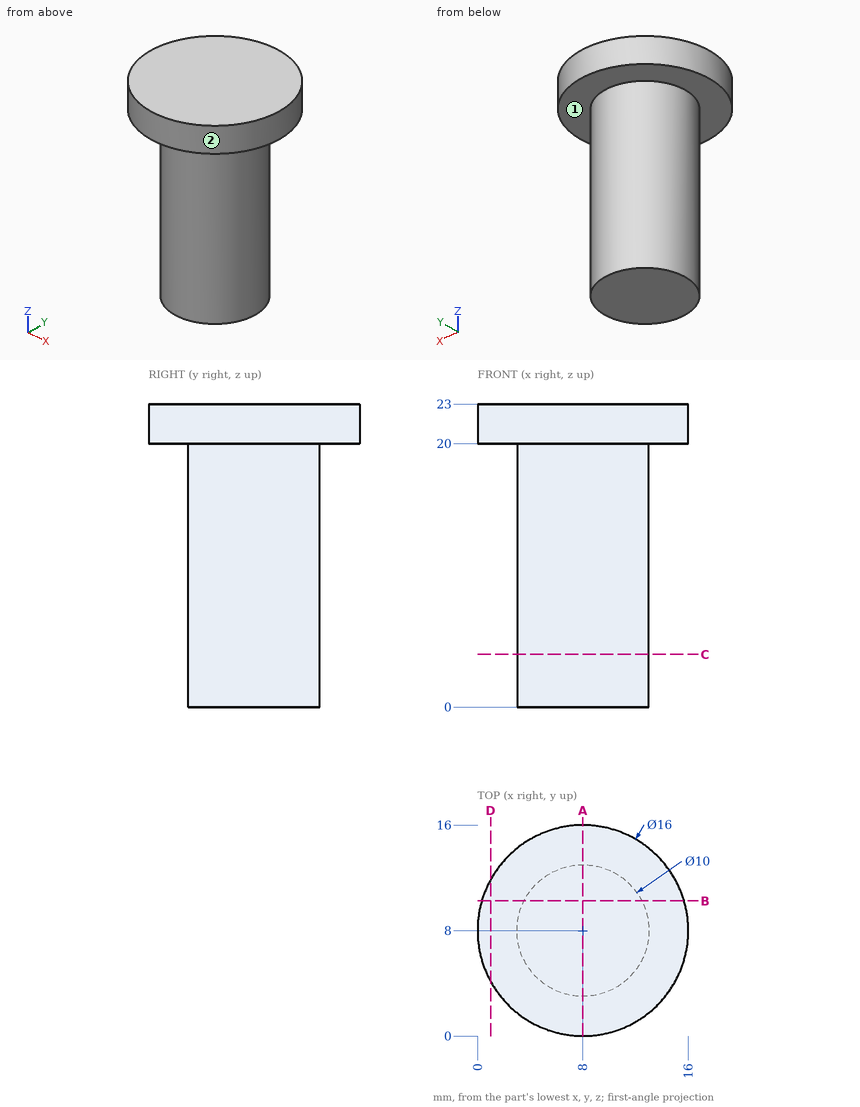
Can you work these out from the drawing? Everything is in mm from the part's minimum corner. A direction names the side the tool comes from. Give positions to 0.01 mm unless a question says otherwise; leave off trailing zeros. Loops run counter-clockwise (first coordinate to the right, second up) from the corner with the lowest first, then second, coordinate; pieces in that order, holes last. Notation, with made-up numbers: (44, 79.5) -> (95, 79.5) arc R14 cw to (95, 88.5) -> close; hole circle Ø11 at (54.25, 57.25). An arc over 180 degrees is marked (long way). Return JSON: item names as keys, results as strings.
Q1. I want a section at C-C, the plane z = 4. List the corners of the cut face in (x, y) for me, then the cut area to 3 significant figures.
Checks:
{"outline": "circle Ø10 at (8, 8)", "area": "78.5 mm2"}
Q2. I need wall thicknesses on probe 1 along Z at (x, y) = (1, 9); probe 2 along X at (y, z) = (7.75, 1.5); probe 3 along X at (y, z) = (4.5, 15). Which ranges of each line are inside material? Lowest first, please.
Checks:
{"probe 1": "z = 20 to 23", "probe 2": "x = 3.01 to 12.99", "probe 3": "x = 4.43 to 11.57"}
Q3. On a 3-axis mill with a long thin cutter (end or side, diameter ignored), from which of +Z, -Z, +X, -X, +Y, -Y can I reach the whole of each face in a straight line? I mean the marked faces 1 and 2. Say none if no direction works.
Checks:
{"face 1": "-Z", "face 2": "+Z, -Z"}
Q4. For pin 1 Ø5 at (x, y) = (9.5, 11) entering from -Z; pin 2 Ø1.5 at (y, z) = (4.5, 14) entering from +X; pin 3 Ø5 at (y, z) = (14.5, 18) entering from +X (3 decimals); pin 4 Ø2 at (y, z) = (4.5, 18.5) entering from +X, each with a flat end and sliding along its axis, tell me the tip position at first contact or that it passes through.
Checks:
{"pin 1": "stops at z = 0", "pin 2": "stops at x = 12.18", "pin 3": "stops at x = 14.245", "pin 4": "stops at x = 12.33"}
Q5. I want a section at A-A, the plane x = 8. List the corners of the cut face in (y, z) for me.
Checks:
{"outline": "(0, 20) -> (3, 20) -> (3, 0) -> (13, 0) -> (13, 20) -> (16, 20) -> (16, 23) -> (0, 23) -> close"}
Q6. I want a section at B-B, the plane y = 10.25. List the corners of the cut face in (x, z) for me, then the cut area to 3 significant figures.
Checks:
{"outline": "(0.32, 20) -> (3.53, 20) -> (3.53, 0) -> (12.47, 0) -> (12.47, 20) -> (15.68, 20) -> (15.68, 23) -> (0.32, 23) -> close", "area": "225 mm2"}
Q7. I want a section at D-D, the plane x = 1. List the corners of the cut face in (y, z) for me.
Checks:
{"outline": "(4.13, 20) -> (11.87, 20) -> (11.87, 23) -> (4.13, 23) -> close"}
